Autodesk Inventor part; units mm, degrees
ref_plane "YZ Plane" through (0, 0, 0) normal (1, 0, 0) x (0, 1, 0)
ref_plane "XZ Plane" through (0, 0, 0) normal (0, 1, 0) x (-1, 0, 0)
ref_plane "XY Plane" through (0, 0, 0) normal (0, 0, 1) x (1, 0, 0)
sketch "Szkic1" plane through (0, 0, 0) normal (0, 1, 0) x (-1, 0, 0)
  line L0 (0, 0) -> (50, 0)
  line L1 (50, 0) -> (50, -50)
  line L2 (50, -50) -> (0, -50)
  line L3 (0, -50) -> (0, 0)
  dimension "d0" = 50
  dimension "d1" = 50
extrude "Wyciągnięcie proste1" add sketch "Szkic1" along normal blind 1.6
sketch "Szkic2" plane through (-50, 0, 0) normal (0, 0, 1) x (1, 0, 0)
  line L0 (0, 0) -> (50, 0)
  line L1 (50, 0) -> (50, 1.6)
  line L2 (0, 1.6) -> (50, 1.6)
  line L3 (0, 0) -> (0, 1.6)
  line L4 (47.9294, 17.85) -> (42.5705, -2.15)
  line L5 (42.5705, -2.15) -> (44.641, -2.15)
  line L6 (44.641, -2.15) -> (50, 17.85)
  line L7 (50, 17.85) -> (47.9294, 17.85)
  point P0 (43.5753, 1.6)
  point P1 (43.1466, 0)
extrude "Wyciągnięcie proste2" cut sketch "Szkic2" against normal through all contours L4 L2 L6 L0 | L6 L2 L1 L0
sketch "Szkic3" plane through (0, 0, 0) normal (0, -1, 0) x (1, 0, 0)
  line L0 (-8.5941, -2) -> (-8.5941, -12.7)
  line L1 (-8.5941, -2) -> (-10.1396, -2)
  line L2 (-10.1396, -12.7) -> (-10.1396, -2)
  line L3 (-8.5941, -12.7) -> (-10.1396, -12.7)
  line L4 (-10.1396, -12.7) -> (-7.8396, -12.7)
  line L5 (-7.8396, -12.7) -> (-7.8396, -2)
  line L6 (-7.8396, -2) -> (-10.1396, -2)
  line L7 (-10.1396, -2) -> (-10.1396, -12.7)
  line L8 (-8.5941, -33) -> (-8.5941, -43.7)
  line L9 (-8.5941, -33) -> (-10.1396, -33)
  line L10 (-10.1396, -43.7) -> (-10.1396, -33)
  line L11 (-8.5941, -43.7) -> (-10.1396, -43.7)
  line L12 (-10.1396, -33) -> (-7.8396, -33)
  line L13 (-7.8396, -33) -> (-7.8396, -43.7)
  line L14 (-7.8396, -43.7) -> (-10.1396, -43.7)
  line L15 (-10.1396, -43.7) -> (-10.1396, -33)
  point P0 (0, 0)
  dimension "d6" = 2.3
  dimension "d7" = 2.3
extrude "Wyciągnięcie proste3" cut sketch "Szkic3" against normal through all
sketch "Szkic4" plane through (0, 0, 0) normal (0, -1, 0) x (1, 0, 0)
  line L0 (-10.1396, -33) -> (-7.8396, -33)
  line L1 (-7.8396, -12.7) -> (-10.1396, -12.7)
  line L2 (-8.9896, -12.7) -> (-8.9896, -33) construction
  circle A0 centre (-8.9896, -26.66) radius 0.55
  circle A1 centre (-8.9896, -24.12) radius 0.55
  circle A2 centre (-8.9896, -21.58) radius 0.55
  circle A3 centre (-8.9896, -19.04) radius 0.55
  point P0 (0, 0)
  dimension "d10" = 1.1
  dimension "d14" = 2.54
  dimension "d19" = 6.34
extrude "Wyciągnięcie proste4" cut sketch "Szkic4" against normal through all
sketch "Szkic5" plane through (0, 0, 0) normal (0, -1, 0) x (1, 0, 0)
  line L0 (-50, -50) -> (-50, 0)
  circle A0 centre (-8.9896, -21.58) radius 0.55
  circle A1 centre (-8.9896, -24.12) radius 0.55
  circle A2 centre (-8.9896, -19.04) radius 0.55
  circle A3 centre (-8.9896, -26.66) radius 0.55
  line L1 (-10.1396, -12.7) -> (-10.1396, -2)
  line L2 (-10.1396, -2) -> (-7.8396, -2)
  line L3 (-7.8396, -2) -> (-7.8396, -12.7)
  line L4 (-7.8396, -12.7) -> (-10.1396, -12.7)
  line L5 (-10.1396, -43.7) -> (-10.1396, -33)
  line L6 (-10.1396, -33) -> (-7.8396, -33)
  line L7 (-7.8396, -33) -> (-7.8396, -43.7)
  line L8 (-7.8396, -43.7) -> (-10.1396, -43.7)
  line L9 (-6.8534, -50) -> (-6.8534, 0)
  line L10 (-50, 0) -> (-6.8534, 0)
  line L11 (-50, -50) -> (-50, 0)
  line L12 (-6.8534, -50) -> (-50, -50)
  line L13 (-50, -50) -> (-50, 0)
  line L14 (-50, -25) -> (-6.8534, -25)
  line L15 (-34, -48.25) -> (-34, -43.25)
  line L16 (-32, -48.25) -> (-34, -48.25)
  line L17 (-32, -43.25) -> (-32, -48.25)
  line L18 (-34, -43.25) -> (-32, -43.25)
  line L19 (-30.5, -46.7732) -> (-30.5, -50)
  line L20 (-36, -50) -> (-50, -50)
  line L21 (-28, -36) -> (-45.016, -36)
  line L22 (-30.5, -50) -> (-36, -50)
  line L23 (-36, -50) -> (-36, -41.75)
  line L24 (-36, -41.75) -> (-30.5, -41.75)
  line L25 (-30.5, -41.75) -> (-30.5, -50)
  line L26 (-36, 0) -> (-36, -8.25)
  line L27 (-36, -8.25) -> (-30.5, -8.25)
  line L28 (-30.5, -8.25) -> (-30.5, 0)
  point P0 (0, 0)
  dimension "d22" = 2
  dimension "d23" = 1.5
extrude "Wyciągnięcie proste5" cut sketch "Szkic5" against normal through all contours L23 L24 L25 L19 L12 | L10 L28 L27 L26 | L15 L18 L17 L16
fillet "Zaokrąglenie2" radius 0.5 2 edges at (-50, 0.8, 0) (-50, 0.8, -50)
sketch "Szkic7" plane through (-6.8534, 0, -50) normal (0, 0, -1) x (-1, 0, 0)
  line L0 (-0.4287, 1.6) -> (23.6466, 1.6)
  line L1 (-0.4287, 1.6) -> (0, 0)
  line L2 (0, 0) -> (23.6466, 0)
  line L3 (0, 0) -> (0, 1.6)
  line L4 (0.2, 1.6) -> (0.2, 0)
  line L5 (23.6466, 0) -> (23.6466, 1.6)
  line L6 (42.6466, 1.6) -> (42.6466, 0)
  line L7 (29.1466, 1.6) -> (42.6466, 1.6)
  line L8 (29.1466, 1.6) -> (29.1466, 0)
  line L9 (29.1466, 0) -> (42.6466, 0)
  point P0 (-6.8534, 0)
  dimension "d30" = 0.2
extrude "Wyciągnięcie proste7" cut sketch "Szkic7" against normal through all contours L0 L3 L1 | L0 L4 L2 L3
sketch "Szkic9" plane through (0, 1.6, 0) normal (0, 1, 0) x (1, 0, 0)
  circle A0 centre (-8.9896, 21.58) radius 0.55
  circle A1 centre (-8.9896, 24.12) radius 0.55
  circle A2 centre (-8.9896, 19.04) radius 0.55
  circle A3 centre (-8.9896, 26.66) radius 0.55
  line L0 (-10.1396, 2) -> (-10.1396, 12.7)
  line L1 (-10.1396, 12.7) -> (-7.8396, 12.7)
  line L2 (-7.8396, 12.7) -> (-7.8396, 2)
  line L3 (-7.8396, 2) -> (-10.1396, 2)
  line L4 (-10.1396, 33) -> (-10.1396, 43.7)
  line L5 (-10.1396, 43.7) -> (-7.8396, 43.7)
  line L6 (-7.8396, 43.7) -> (-7.8396, 33)
  line L7 (-7.8396, 33) -> (-10.1396, 33)
  line L8 (-7.0534, 0) -> (-7.0534, 50)
  line L9 (-7.0534, 50) -> (-30.5, 50)
  line L10 (-30.5, 50) -> (-30.5, 41.75)
  line L11 (-30.5, 41.75) -> (-36, 41.75)
  line L12 (-36, 41.75) -> (-36, 50)
  line L13 (-36, 50) -> (-49.5, 50)
  arc A4 (-49.5, 50) -> (-50, 49.5) centre (-49.5, 49.5) ccw
  line L14 (-50, 49.5) -> (-50, 0.5)
  arc A5 (-50, 0.5) -> (-49.5, 0) centre (-49.5, 0.5) ccw
  line L15 (-49.5, 0) -> (-36, 0)
  line L16 (-36, 0) -> (-36, 8.25)
  line L17 (-36, 8.25) -> (-30.5, 8.25)
  line L18 (-30.5, 8.25) -> (-30.5, 0)
  line L19 (-30.5, 0) -> (-7.0534, 0)
  line L20 (-10.1396, 12.7) -> (-7.0534, 12.7)
  line L21 (-7.0534, 12.7) -> (-7.0534, 2)
  line L22 (-7.0534, 2) -> (-10.1396, 2)
  line L23 (-10.1396, 2) -> (-10.1396, 12.7)
  line L24 (-10.1396, 43.7) -> (-7.0534, 43.7)
  line L25 (-7.0534, 43.7) -> (-7.0534, 33)
  line L26 (-7.0534, 33) -> (-10.1396, 33)
  line L27 (-10.1396, 33) -> (-10.1396, 43.7)
  point P0 (0, 0)
  point P1 (-7.8396, 2)
extrude "Wyciągnięcie proste8" cut sketch "Szkic9" against normal through all contours L2 L20 L8 L22 | L26 L6 L24 L8
fillet "Zaokrąglenie3" radius 0.5 6 edges at (-7.0534, 0.8, -12.7) (-7.0534, 0.8, -33) (-7.0534, 0.8, -43.7) (-7.0534, 0.8, -50) (-7.0534, 0.8, -2) (-7.0534, 0.8, 0)
sketch "Szkic11" plane through (0, 0, 0) normal (0, -1, 0) x (1, 0, 0)
  arc A0 (-7.0534, -0.5) -> (-7.5534, 0) centre (-7.5534, -0.5) ccw
  line L0 (-30.5, 0) -> (-7.5534, 0)
  line L1 (-30.5, 0) -> (-30.5, -8.25)
  line L2 (-30.5, -8.25) -> (-36, -8.25)
  line L3 (-36, -8.25) -> (-36, 0)
  line L4 (-49.5, 0) -> (-36, 0)
  arc A1 (-49.5, 0) -> (-50, -0.5) centre (-49.5, -0.5) ccw
  line L5 (-50, -49.5) -> (-50, -0.5)
  arc A2 (-50, -49.5) -> (-49.5, -50) centre (-49.5, -49.5) ccw
  line L6 (-36, -50) -> (-49.5, -50)
  line L7 (-36, -50) -> (-36, -41.75)
  line L8 (-36, -41.75) -> (-30.5, -41.75)
  line L9 (-30.5, -41.75) -> (-30.5, -50)
  line L10 (-7.5534, -50) -> (-30.5, -50)
  arc A3 (-7.5534, -50) -> (-7.0534, -49.5) centre (-7.5534, -49.5) ccw
  line L11 (-7.0534, -49.5) -> (-7.0534, -44.2)
  arc A4 (-7.0534, -44.2) -> (-7.5534, -43.7) centre (-7.5534, -44.2) ccw
  line L12 (-7.5534, -43.7) -> (-10.1396, -43.7)
  line L13 (-10.1396, -43.7) -> (-10.1396, -33)
  line L14 (-10.1396, -33) -> (-7.5534, -33)
  arc A5 (-7.5534, -33) -> (-7.0534, -32.5) centre (-7.5534, -32.5) ccw
  line L15 (-7.0534, -32.5) -> (-7.0534, -13.2)
  arc A6 (-7.0534, -13.2) -> (-7.5534, -12.7) centre (-7.5534, -13.2) ccw
  line L16 (-7.5534, -12.7) -> (-10.1396, -12.7)
  line L17 (-10.1396, -12.7) -> (-10.1396, -2)
  line L18 (-10.1396, -2) -> (-7.5534, -2)
  arc A7 (-7.5534, -2) -> (-7.0534, -1.5) centre (-7.5534, -1.5) ccw
  line L19 (-7.0534, -1.5) -> (-7.0534, -0.5)
  circle A8 centre (-8.9896, -26.66) radius 0.55
  circle A9 centre (-8.9896, -19.04) radius 0.55
  circle A10 centre (-8.9896, -24.12) radius 0.55
  circle A11 centre (-8.9896, -21.58) radius 0.55
  line L20 (-30.5, 0) -> (-31, 0)
  line L21 (-31, 0) -> (-31, -8.25)
  line L22 (-31, -8.25) -> (-30.5, -8.25)
  line L23 (-30.5, -8.25) -> (-30.5, 0)
  line L24 (-30.5, -50) -> (-31, -50)
  line L25 (-31, -50) -> (-31, -41.75)
  line L26 (-31, -41.75) -> (-30.5, -41.75)
  line L27 (-30.5, -41.75) -> (-30.5, -50)
  point P0 (0, 0)
  dimension "d40" = 0.5
  dimension "d41" = 0.5
extrude "Wyciągnięcie proste10" add sketch "Szkic11" against normal up to surface (1.6 mm away) contours L1 L2 L21 L20 | L8 L9 L24 L25
fillet "Zaokrąglenie4" radius 1.5 2 edges at (-31, 0.8, -50) (-31, 0.8, 0)
fillet "Zaokrąglenie5" radius 0.5 6 edges at (-31, 0.8, -8.25) (-36, 0.8, -8.25) (-36, 0.8, 0) (-36, 0.8, -50) (-36, 0.8, -41.75) (-31, 0.8, -41.75)
sketch "Szkic13" plane through (0, 0, 0) normal (0, -1, 0) x (1, 0, 0)
  circle A0 centre (-28.5, -2.5) radius 1
  circle A1 centre (-28.5, -47.5) radius 1
  point P0 (0, 0)
hole "Otwór2" at (-28.5, 0, -2.5) at (-28.5, 0, -47.5) direction (0, 1, 0) diameter 2.6 end through all
fillet "Zaokrąglenie6" radius 0.5 1 edges at (-28.5, 1.6, -1.2)
sketch "Szkic14" plane through (0, 0, 0) normal (0, -1, 0) x (1, 0, 0)
  circle A0 centre (-28.5, -2.5) radius 1.3
  circle A1 centre (-28.5, -47.5) radius 1.3
  arc A2 (-36.5, -50) -> (-36, -49.5) centre (-36.5, -49.5) ccw
  line L0 (-36, -49.5) -> (-36, -42.25)
  arc A3 (-35.5, -41.75) -> (-36, -42.25) centre (-35.5, -42.25) ccw
  line L1 (-35.5, -41.75) -> (-31.5, -41.75)
  arc A4 (-31, -42.25) -> (-31.5, -41.75) centre (-31.5, -42.25) ccw
  line L2 (-31, -42.25) -> (-31, -48.5)
  arc A5 (-31, -48.5) -> (-29.5, -50) centre (-29.5, -48.5) ccw
  line L3 (-29.5, -50) -> (-7.5534, -50)
  arc A6 (-7.5534, -50) -> (-7.0534, -49.5) centre (-7.5534, -49.5) ccw
  line L4 (-7.0534, -49.5) -> (-7.0534, -44.2)
  arc A7 (-7.0534, -44.2) -> (-7.5534, -43.7) centre (-7.5534, -44.2) ccw
  line L5 (-7.5534, -43.7) -> (-10.1396, -43.7)
  line L6 (-10.1396, -43.7) -> (-10.1396, -33)
  line L7 (-10.1396, -33) -> (-7.5534, -33)
  arc A8 (-7.5534, -33) -> (-7.0534, -32.5) centre (-7.5534, -32.5) ccw
  line L8 (-7.0534, -32.5) -> (-7.0534, -13.2)
  arc A9 (-7.0534, -13.2) -> (-7.5534, -12.7) centre (-7.5534, -13.2) ccw
  line L9 (-7.5534, -12.7) -> (-10.1396, -12.7)
  line L10 (-10.1396, -12.7) -> (-10.1396, -2)
  line L11 (-10.1396, -2) -> (-7.5534, -2)
  arc A10 (-7.5534, -2) -> (-7.0534, -1.5) centre (-7.5534, -1.5) ccw
  line L12 (-7.0534, -1.5) -> (-7.0534, -0.5)
  arc A11 (-7.0534, -0.5) -> (-7.5534, 0) centre (-7.5534, -0.5) ccw
  line L13 (-29.5, 0) -> (-7.5534, 0)
  arc A12 (-29.5, 0) -> (-31, -1.5) centre (-29.5, -1.5) ccw
  line L14 (-31, -1.5) -> (-31, -7.75)
  arc A13 (-31.5, -8.25) -> (-31, -7.75) centre (-31.5, -7.75) ccw
  line L15 (-31.5, -8.25) -> (-35.5, -8.25)
  arc A14 (-36, -7.75) -> (-35.5, -8.25) centre (-35.5, -7.75) ccw
  line L16 (-36, -7.75) -> (-36, -0.5)
  arc A15 (-36, -0.5) -> (-36.5, 0) centre (-36.5, -0.5) ccw
  line L17 (-49.5, 0) -> (-36.5, 0)
  arc A16 (-49.5, 0) -> (-50, -0.5) centre (-49.5, -0.5) ccw
  line L18 (-50, -49.5) -> (-50, -0.5)
  arc A17 (-50, -49.5) -> (-49.5, -50) centre (-49.5, -49.5) ccw
  line L19 (-36.5, -50) -> (-49.5, -50)
  circle A18 centre (-8.9896, -21.58) radius 0.55
  circle A19 centre (-8.9896, -24.12) radius 0.55
  circle A20 centre (-8.9896, -19.04) radius 0.55
  circle A21 centre (-8.9896, -26.66) radius 0.55
  point P0 (0, 0)
properties part number "PCB_GORNE"
Here's how the part is built. I have some questions about the finished solid (model axes, mm). A direction names the side the tool comes from. Give positions to 0.01 mm unless a question says otherwise; leave off trailing zeros. Order: outer loops, then holes, each group sorted by start corner. A loop starts at its lowest first (then second) coordinate and runs counter-clockwise, first axis right, second up. Notation, with made-up numbers: (78, 21.25) -> (107, 21.25) arc R18 cw to (107, 54.25) -> close; hole circle Ø11 at (-37, 47). An arc over 180 degrees is marked (long way). Use a Markdown table: item, result. Add a question column.
Item 1: Will these pins go through, and if not, where does the flat tip stop? pin 1 (1 mm diameter, centred on x = -8.99, z = -19.04, fed in from -Y); pin 2 (0.8 mm diameter, centred on y = 1, z = -8, fed in from +X).
Item 2: Imagine slicing it at C-C on z = -21.58. Please give me the cut outline in (x, y), plus the area to 3 significant figures.
Item 3: For faces 4 (the face through (-34, 1, -41.75)), 5 (the face through (-34, 1, -8.25)), 6 (the face through (-9.43, 0.79, -21.91)), 7 (the face through (-9, 1, -43.7)), which set-ups out of +Z, -Z, +X, -X, +Y, -Y let a thin tool reach every point of the face, with its end or its side?
Item 4: Imagine slicing it at A-A on z = -47.5. Please give me the cut outline in (x, y).
Item 5: If we mould it in two halves opening along X, with no side actions, what happens to faces 1 (the face through (-9, 1, -33)), 2 (the face through (-10.14, 1, -7)), 3 (the face through (-30.55, 0.81, -49.57))? For each: pulls with the +X half, pulls with the -X half, needs draft (parallel to the pull), parting line crosses it, or undercut.
Item 6: Imagine slicing it at D-D on z = -6. Please give me the cut outline in (x, y), plus the area to 3 significant figures.
Item 7: I need wall thicknesses on line 1 (Z direction, x = -28.5, y = 1.05); line 2 (X direction, y = 0.3, z = -2.5); line 3 (X direction, y = 0.35, z = -6.5). Which ranges of each line are inside material? Lowest first, please.
Item 8: Imagine slicing it at B-B on x = -28.5. Please give me the cut outline in (y, z), plus the area to 3 significant figures.
Data:
| question | item | result |
|---|---|---|
| 1 | pin 1 | passes through |
| 1 | pin 2 | stops at x = -10.14 |
| 2 | outline | (-50, 0) -> (-9.54, 0) -> (-9.54, 1.6) -> (-50, 1.6) -> close; (-8.44, 0) -> (-7.05, 0) -> (-7.05, 1.6) -> (-8.44, 1.6) -> close |
| 2 | area | 67.0 mm² |
| 3 | face 4 | -Z, +Y, -Y |
| 3 | face 5 | +Z, +Y, -Y |
| 3 | face 6 | +Y, -Y |
| 3 | face 7 | +X, +Y, -Y |
| 4 | outline | (-50, 0) -> (-36, 0) -> (-36, 1.6) -> (-50, 1.6) -> close; (-31, 0) -> (-29.8, 0) -> (-29.8, 1.6) -> (-31, 1.6) -> close; (-27.2, 0) -> (-7.05, 0) -> (-7.05, 1.6) -> (-27.2, 1.6) -> close |
| 5 | face 1 | needs draft |
| 5 | face 2 | pulls with the +X half |
| 5 | face 3 | undercut |
| 6 | outline | (-50, 0) -> (-36, 0) -> (-36, 1.6) -> (-50, 1.6) -> close; (-31, 0) -> (-10.14, 0) -> (-10.14, 1.6) -> (-31, 1.6) -> close |
| 6 | area | 55.8 mm² |
| 7 | line 1 | z = -50 to -48.8, -46.2 to -3.8, -1.2 to 0 |
| 7 | line 2 | x = -50 to -36, -31 to -29.8, -27.2 to -10.14 |
| 7 | line 3 | x = -50 to -36, -31 to -10.14 |
| 8 | outline | (0, -50) -> (1.6, -50) -> (1.6, -48.8) -> (0, -48.8) -> close; (0, -46.2) -> (1.6, -46.2) -> (1.6, -4.3) arc R0.5 ccw to (1.1, -3.8) -> (0, -3.8) -> close; (0, -1.2) -> (1.1, -1.2) arc R0.5 ccw to (1.6, -0.7) -> (1.6, 0) -> (0, 0) -> close |
| 8 | area | 71.6 mm² |
